from build123d import *

# Parameters (mm, degrees)
F0_R     = 1.55
F1_DEPTH = 2


with BuildPart() as f1:
    # F0 (on Top) → F1 (new body)
    with BuildSketch(Plane.XY):
        with BuildLine():
            Line((24.31838, 19.181142), (24.31838, 33.05))
            ThreePointArc((24.31838, 33.05), (23.000361, 36.231981), (19.81838, 37.55))
            Line((19.81838, 37.55), (-1.037385, 37.55))
            ThreePointArc((-1.037385, 37.55), (-9.969408, 35.177507), (-16.546857, 28.685441))
            Line((-16.546857, 28.685441), (-21.480482, 20.840884))
            ThreePointArc((-21.480482, 20.840884), (-22.568149, 19.615657), (-23.993472, 18.807786))
            Line((-23.993472, 18.807786), (-46.541382, 10.54976))
            ThreePointArc((-46.541382, 10.54976), (-47.730939, 9.634135), (-48.181621, 8.202248))
            Line((-48.181621, 8.202248), (-48.181621, -8.202248))
            ThreePointArc((-48.181621, -8.202248), (-47.730939, -9.634135), (-46.541382, -10.54976))
            Line((-46.541382, -10.54976), (-23.993472, -18.807786))
            ThreePointArc((-23.993472, -18.807786), (-22.568149, -19.615657), (-21.480482, -20.840884))
            Line((-21.480482, -20.840884), (-16.546857, -28.685441))
            ThreePointArc((-16.546857, -28.685441), (-9.969408, -35.177507), (-1.037385, -37.55))
            Line((-1.037385, -37.55), (19.81838, -37.55))
            ThreePointArc((19.81838, -37.55), (23.000361, -36.231981), (24.31838, -33.05))
            Line((24.31838, -33.05), (24.31838, -19.181142))
            ThreePointArc((24.31838, -19.181142), (25.782846, -15.645608), (29.31838, -14.181142))
            Line((29.31838, -14.181142), (35.911883, -14.181142))
            ThreePointArc((35.911883, -14.181142), (39.447417, -12.716676), (40.911883, -9.181142))
            Line((40.911883, -9.181142), (40.911883, 0))
            Line((40.911883, 0), (40.911883, 9.181142))
            ThreePointArc((40.911883, 9.181142), (39.447417, 12.716676), (35.911883, 14.181142))
            Line((35.911883, 14.181142), (29.31838, 14.181142))
            ThreePointArc((29.31838, 14.181142), (25.782846, 15.645608), (24.31838, 19.181142))
        make_face()
        with Locations((-44.231621, -7)):
            Circle(F0_R, mode=Mode.SUBTRACT)
        with Locations((12.81838, -33.05)):
            Circle(F0_R, mode=Mode.SUBTRACT)
        with Locations((19.81838, -33.05)):
            Circle(F0_R, mode=Mode.SUBTRACT)
        with Locations((-44.231621, 7)):
            Circle(F0_R, mode=Mode.SUBTRACT)
        with BuildLine():
            Line((-13.039333, 17.357413), (-7.470524, 26.211925))
            ThreePointArc((-7.470524, 26.211925), (-5.655694, 27.926621), (-3.238012, 28.55))
            Line((-3.238012, 28.55), (10.31838, 28.55))
            ThreePointArc((10.31838, 28.55), (12.439701, 27.67132), (13.31838, 25.55))
            Line((13.31838, 25.55), (13.31838, -25.55))
            ThreePointArc((13.31838, -25.55), (12.439701, -27.67132), (10.31838, -28.55))
            Line((10.31838, -28.55), (-3.238012, -28.55))
            ThreePointArc((-3.238012, -28.55), (-5.655694, -27.926621), (-7.470524, -26.211925))
            Line((-7.470524, -26.211925), (-13.039333, -17.357413))
            ThreePointArc((-13.039333, -17.357413), (-13.839835, -15.569969), (-14.113817, -13.630718))
            Line((-14.113817, -13.630718), (-14.113817, 13.630718))
            ThreePointArc((-14.113817, 13.630718), (-13.839835, 15.569969), (-13.039333, 17.357413))
        make_face(mode=Mode.SUBTRACT)
        with Locations((12.81838, 33.05)):
            Circle(F0_R, mode=Mode.SUBTRACT)
        with Locations((19.81838, 33.05)):
            Circle(F0_R, mode=Mode.SUBTRACT)
    extrude(amount=F1_DEPTH)


solid = f1.part
Check sheet for the modelled part. Datum: model origin and axes. Units: mm. A direction names the side the tool comes from. Give positions to 0.01 mm unless a question says otherwise; leave off trailing zeros. Write each loop counter-clockwise with the first axis right and the second up, starting at its lowest first coordinate (ties: lowest second). Pieces come first, ordered by that corner, then holes. Notation, with made-up numbers: (-32.75, 70.25) -> (-10.75, 70.25) arc R22 ccw to (-10.75, 106.25) -> close; hole circle Ø7 at (50, 11.25). An arc over 180 degrees is marked (long way). Use one line per item in the form item = value. Start each with the question number.
1. Section check B-B (z = 0.5). Count the separate pieces of the cut face and the enclosed holes in it, and give its area (3 significant figures).
2. Section check D-D (x = -40.5). Record the cut outline in (y, z), and give its area (3 significant figures).
3. Go/stop test with flat-tipped pins: P1, Ø1, axis at y = 25.5, z = 1, coming from the +X side; P2, Ø2.5, axis at x = 12.82, y = -33.05, coming from the -Z side; P3, Ø1, axis at x = 34, z = 1.5, coming from the -Y side; P4, Ø0.6, axis at x = 33, z = 1, coming from the +Y side. Record where each tip stops, or that it passes through.
4. Thickness scan on line 1 along Y through (x, z) = (0, 1); line 2 along X through (y, z) = (-2, 1.75); line 3 along X through (y, z) = (33.5, 1.45). Record the ranges inside material, lowest first. Write a range as from..to.
5. Section check A-A (y = -2). Record the cut outline in (x, z).
6. Access from +Z, -Z, +X, -X, +Y, -Y to the whole of each face (thin tool, end or side, straight path). Record for faces 1 (the flat face through (33, 14.181, 1)), 2 (the flat face through (3, 28.55, 1)), 3 (the flat face through (16, 1, 0)).
7. Section check C-C (y = -12.5). Record the cut outline in (x, z), and give its area (3 significant figures).
Conclusion:
q1.separate_pieces = 1
q1.enclosed_holes = 7
q1.area = 2,990 mm²
q2.outline = (-12.76, 0) -> (12.76, 0) -> (12.76, 2) -> (-12.76, 2) -> close
q2.area = 51.0 mm²
q3.P1 = 24.32
q3.P2 = through
q3.P3 = -14.18
q3.P4 = 14.18
q4.line_1 = -37.55..-28.55, 28.55..37.55
q4.line_2 = -48.18..-14.11, 13.32..40.91
q4.line_3 = -12.41..11.34, 14.3..18.34, 21.3..24.3
q5.outline = (-48.18, 0) -> (-14.11, 0) -> (-14.11, 2) -> (-48.18, 2) -> close; (13.32, 0) -> (40.91, 0) -> (40.91, 2) -> (13.32, 2) -> close
q6.face_1 = +Z, -Z, +X, +Y
q6.face_2 = +Z, -Z
q6.face_3 = -Z, +X, -X, +Y, -Y
q7.outline = (-41.22, 0) -> (-14.11, 0) -> (-14.11, 2) -> (-41.22, 2) -> close; (13.32, 0) -> (39.65, 0) -> (39.65, 2) -> (13.32, 2) -> close
q7.area = 107 mm²
